Verification items for the finished model (mm, model axes). Face numbers are marked on the shaded views. Round coordinates to 2 decimals unless told otherwise and drop trailing zeros. Loops run counter-clockwise (first coordinate to the right, second up) from the corner with the lowest first, then second, coordinate; pieces in that order, holes last. Notation, with made-up numbers: (14.25, 43) - (46.25, 43) arc R20 cw to (46.25, 61) - close; hole circle Ø10 at (54, 82.5). An arc over 180 degrees is marked (long way). Use CSV: the item, a comma, the result in double quotes.
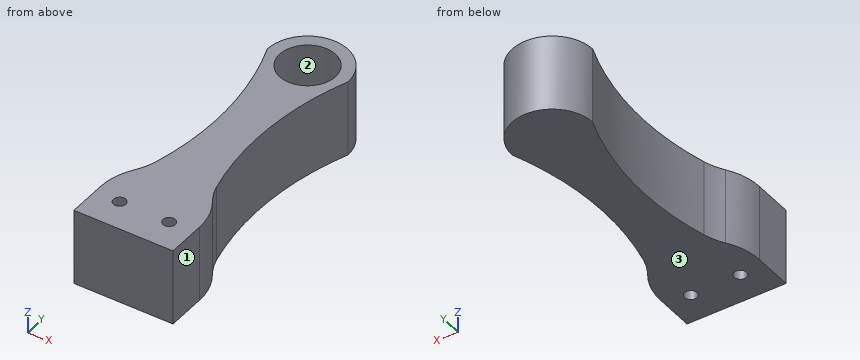
Autodesk Inventor part; units mm, degrees
ref_plane "YZ Plane" through (0, 0, 0) normal (1, 0, 0) x (0, 1, 0)
ref_plane "XZ Plane" through (0, 0, 0) normal (0, 1, 0) x (-1, 0, 0)
ref_plane "XY Plane" through (0, 0, 0) normal (0, 0, 1) x (1, 0, 0)
sketch "Sketch1" plane through (0, 0, 0) normal (0, 1, 0) x (-1, 0, 0)
  line L0 (0, 0) -> (16, 0)
  line L1 (16, 0) -> (16, -12.3)
  line L2 (16, -12.3) -> (0, -12.3)
  line L3 (0, -12.3) -> (0, 0)
  dimension "d0" = 16
  dimension "d1" = 12.3
extrude "Extrusion1" add sketch "Sketch1" along normal blind 10
sketch "Sketch2" plane through (0, 10, 0) normal (0, 1, 0) x (1, 0, 0)
  line L0 (-16, 0) -> (0, 0)
  line L1 (-8, 0) -> (-8, 12.3)
  line L2 (0, 12.3) -> (-16, 12.3)
  line L3 (-14.5, 0) -> (-14.5, 12.3)
  line L4 (-1.5, 0) -> (-1.5, 12.3)
  dimension "d4" = 6.5
  dimension "d5" = 6.5
extrude "Extrusion2" add sketch "Sketch2" along normal blind 40.5
sketch "Sketch3" plane through (-16, 0, 0) normal (0, 0, 1) x (1, 0, 0)
  line L0 (14.5, 50.5) -> (1.5, 50.5)
  line L1 (8, 50.5) -> (8, 0)
  line L2 (0, 0) -> (16, 0)
  circle A0 centre (8, 44) radius 4.5
  line L3 (1.5, 50.5) -> (14.5, 50.5)
  circle A1 centre (8, 44) radius 6.5
  line L4 (14.5, 10) -> (14.5, 50.5)
  line L5 (14.5, 30.25) -> (1.5, 30.25)
  line L6 (1.5, 10) -> (1.5, 50.5)
  line L7 (8, 30.25) -> (11.5, 30.25)
  arc A2 (14.5, 44) -> (14.5, 10) centre (59.4062, 27) ccw
  line L8 (8, 30.25) -> (4.5, 30.25)
  arc A3 (1.5, 10) -> (1.5, 44) centre (-43.4062, 27) ccw
  dimension "d8" = 6.5
  dimension "d9" = 9
  dimension "d10" = 13
  dimension "d11" = 3.5
  dimension "d12" = 3.5
extrude "Extrusion3" cut sketch "Sketch3" against normal blind 13.5 contours L4 A1 L0 | A1 L6 L0 | L4 L5 A2 A1 | A1 A2 | A3 A1 | A1 A3 L5 L6 | L4 A2 L5 | L5 A3 L6
fillet "Fillet1" radius 10 4 edges at (0, 10, -6.15) (-1.5, 10, -6.15) (-14.5, 10, -6.15) (-16, 10, -6.15)
sketch "Sketch4" plane through (-16, 0, 0) normal (0, 0, 1) x (1, 0, 0)
  arc A0 (14.5, 44) -> (1.5, 44) centre (8, 44) ccw
  circle A1 centre (8, 44) radius 4.5
  point P0 (16, 0)
  dimension "d16" = 9
extrude "Extrusion4" cut sketch "Sketch4" against normal blind 8.23
sketch "Sketch5" plane through (0, 0, 0) normal (0, -1, 0) x (1, 0, 0)
  point P0 (0, 0)
sketch "Sketch7" plane through (-16, 0, 0) normal (0, 0, 1) x (1, 0, 0)
  line L0 (16, 0) -> (0, 0)
  line L1 (0, 0) -> (16, 0)
  line L2 (16, 0) -> (16, 10)
  line L3 (16, 10) -> (0, 10)
  line L4 (0, 10) -> (0, 0)
  line L5 (0, 5) -> (16, 5)
  line L6 (8, 10) -> (8, 0)
  circle A0 centre (4, 5) radius 1
  circle A1 centre (12, 5) radius 1
extrude "Extrusion6" cut sketch "Sketch7" against normal blind 12.3 contours A1 L5 | L5 A1 | A0 L5 | L5 A0
properties part number "pawn"
1) Gauge pin test, flat ends, axial feed: pin 1 Ø2 at (y, z) = (21.5, -4) entering from +X; pin 2 Ø1.5 at (y, z) = (17, -9) entering from +X; pin 3 Ø3 at (y, z) = (27, -9) entering from +X. Record the tip position at first contact, or that the pin passes through.
Returned:
pin 1,"stops at x = -4.17"
pin 2,"stops at x = -3.39"
pin 3,"stops at x = -4.59"
2) Cross-section at A-A, the plane z = -9.5. Record the cut outline in (x, y).
Returned:
outline,"(-16, 0) - (0, 0) - (0, 6.35) arc R10 ccw to (-1.7, 11.94) arc R10 cw to (-3.09, 15.03) arc R48.02 cw to (-1.5, 44) arc R6.5 ccw to (-14.5, 44) arc R48.02 cw to (-12.91, 15.03) arc R10 cw to (-14.3, 11.94) arc R10 ccw to (-16, 6.35) - close; hole circle Ø2 at (-12, 5); hole circle Ø2 at (-4, 5)"
3) Thickness scan on probe 1 along Y at (x, z) = (-8, -5.5); probe 2 along X at (y, z) = (5, -5.75); probe 3 along Y at (x, z) = (-10.75, -5.75). Record the ranges inside material, lowest first. Write a range as [from, to].
Returned:
probe 1,"y = [0, 39.5], [48.5, 50.5]"
probe 2,"x = [-16, -13], [-11, -5], [-3, 0]"
probe 3,"y = [0, 40.44], [47.56, 49.89]"
4) Cross-section at C-C, the plane x = -8. Record the cut outline in (y, z).
Returned:
outline,"(0, -12.3) - (50.5, -12.3) - (50.5, 0) - (48.5, 0) - (48.5, -8.23) - (39.5, -8.23) - (39.5, 0) - (0, 0) - close"
5) Cross-section at B-B, the plane y = 5. Record the cut outline in (x, z).
Returned:
outline,"(-16, -12.3) - (-13, -12.3) - (-13, 0) - (-16, 0) - close; (-11, -12.3) - (-5, -12.3) - (-5, 0) - (-11, 0) - close; (-3, -12.3) - (0, -12.3) - (0, 0) - (-3, 0) - close"
6) Mould release check, pull along X, two halves, no side actions. Record for the marked faces 1, 2 and 3: +X half, -X half, draft (parallel to the pull), parting line (faces both ways), or undercut.
Returned:
face 1,"+X half"
face 2,"undercut"
face 3,"draft"
7) Cross-section at D-D, the plane x = -4. Record the cut outline in (y, z).
Returned:
outline,"(0, -12.3) - (4, -12.3) - (4, 0) - (0, 0) - close; (6, -12.3) - (19.37, -12.3) - (19.37, 0) - (6, 0) - close; (34.63, -12.3) - (49.12, -12.3) - (49.12, 0) - (46.06, 0) - (46.06, -8.23) - (41.94, -8.23) - (41.94, 0) - (34.63, 0) - close"
